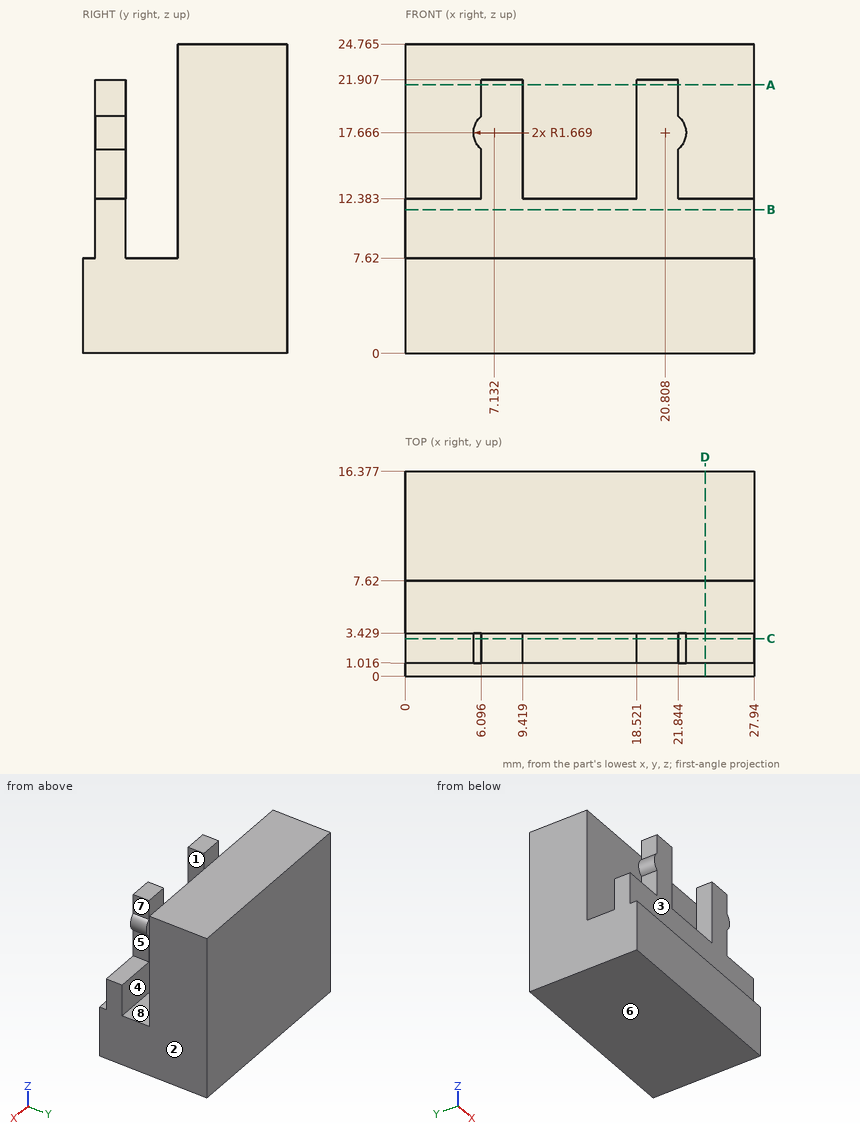
Check sheet for the drawn part. Datum: minimum x, y, z corner. Units: mm. A direction names the side the tool comes from. Round coordinates to 2 decimals unless told otherwise and drop trailing zeros. Loops run counter-clockwise (first coordinate to the right, second up) from the corner with the lowest first, then second, coordinate; pieces in that order, holes last. Notation, with made-up numbers: (89.25, 35.5) -> (116.25, 35.5) arc R32 ccw to (116.25, 70.5) -> close; hole circle Ø2 at (83, 29). An arc over 180 degrees is marked (long way). Put each result on its own line as item: value. Start each with the question number.
1. Section check D-D (x = 24). Enter the section's corners in (y, z) (1 decimal).
2. Draft check along Z on the marked faces 5, 6, 7 and 8. Enter one of: +Z half, -Z half, draft (parallel to the pull), parting line (faces both ways), or undercut.
3. Gauge pin test, flat ends, axial feed: pin 1 (2.5 mm diameter, centred on x = 24.5, y = 2, fed in from +Z); pin 2 (0.7 mm diameter, centred on x = 20, y = 2, fed in from +Z); pin 3 (1.2 mm diameter, centred on y = 2, z = 21, fed in from -X). Record the tip position at first contact, or that the pin passes through.
4. Section check B-B (z = 11.5). Enter the section's corners in (x, y) (1 decimal), plus the area to 3 significant figures.
5. Section check C-C (y = 3). Enter the section's corners in (x, z) (1 decimal).
6. Section check A-A (z = 21.5). Enter the section's corners in (x, y) (1 decimal).
7. Scan lines: probe 1 along Y at (x, z) = (22.25, 18) (1 decimal); probe 2 along Z at (x, y) = (24.25, 6); probe 3 along X at (y, z) = (1.75, 14.5) (1 decimal). Record each from-to range of solid material in increasing order.
8. Access from +Z, -Z, +X, -X, +Y, -Y to the whole of each face (thin tool, end or side, straight path). Record for the marked faces 1, 2, 3 and 4.
Findings:
1. outline: (0, 0) -> (16.4, 0) -> (16.4, 24.8) -> (7.6, 24.8) -> (7.6, 7.6) -> (3.4, 7.6) -> (3.4, 12.4) -> (1, 12.4) -> (1, 7.6) -> (0, 7.6) -> close
2. face 5: undercut
2. face 6: -Z half
2. face 7: draft
2. face 8: +Z half
3. pin 1: stops at z = 12.38
3. pin 2: stops at z = 21.91
3. pin 3: stops at x = 6.1
4. outline: (0, 1) -> (27.9, 1) -> (27.9, 3.4) -> (0, 3.4) -> close; (0, 7.6) -> (27.9, 7.6) -> (27.9, 16.4) -> (0, 16.4) -> close
4. area: 312 mm^2
5. outline: (0, 0) -> (27.9, 0) -> (27.9, 12.4) -> (21.8, 12.4) -> (21.8, 16.4) arc R1.7 ccw to (21.8, 19) -> (21.8, 21.9) -> (18.5, 21.9) -> (18.5, 12.4) -> (9.4, 12.4) -> (9.4, 21.9) -> (6.1, 21.9) -> (6.1, 19) arc R1.7 ccw to (6.1, 16.4) -> (6.1, 12.4) -> (0, 12.4) -> close
6. outline: (0, 7.6) -> (27.9, 7.6) -> (27.9, 16.4) -> (0, 16.4) -> close; (6.1, 1) -> (9.4, 1) -> (9.4, 3.4) -> (6.1, 3.4) -> close; (18.5, 1) -> (21.8, 1) -> (21.8, 3.4) -> (18.5, 3.4) -> close
7. probe 1: y = 1 to 3.4, 7.6 to 16.4
7. probe 2: z = 0 to 7.62
7. probe 3: x = 6.1 to 9.4, 18.5 to 21.8
8. face 1: +Z, -Y
8. face 2: +Z, -Z, +X, +Y, -Y
8. face 3: +Z, +X, -X, -Y
8. face 4: +Z, +X, -X
